from build123d import *

# Parameters (mm, degrees)
F1_DEPTH = 2
F2_R     = 1


with BuildPart() as f1:
    # F0 (on Top) → F1 (new body)
    with BuildSketch(Plane.XY):
        with BuildLine():
            ThreePointArc((13.617544, 3.25), (-14, 0), (13.617544, -3.25))
            Line((13.617544, -3.25), (2.436699, -1.75))
            ThreePointArc((2.436699, -1.75), (-3, 0), (2.436699, 1.75))
            Line((2.436699, 1.75), (13.617544, 3.25))
        make_face()
    extrude(amount=F1_DEPTH)

    # F2
    f2_edges = [f1.edges().sort_by_distance(p)[0] for p in [
        (13.617544, 3.25, 1),
        (13.617544, -3.25, 1),
    ]]
    fillet(f2_edges, radius=F2_R)


solid = f1.part
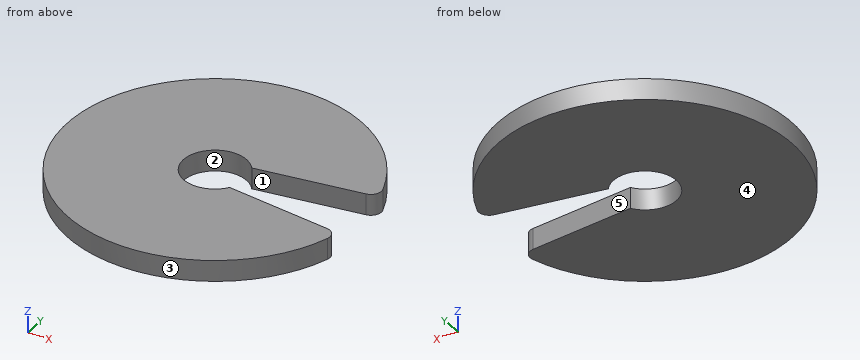
Build history of the part. All positions in model axes, mm. Face numbers are marked on the shaded views. A direction names the side the tool comes from. Give positions to 0.01 mm unless a question says otherwise; leave off trailing zeros. Loops run counter-clockwise (first coordinate to the right, second up) from the corner with the lowest first, then second, coordinate; pieces in that order, holes last. Notation, with made-up numbers: (-27, 27) - (-18, 27) arc R15 ccw to (-18, 43) - close; hole circle Ø4 at (72.25, 82). An arc over 180 degrees is marked (long way). Write item = value, one per line. Start each with the question number.
1) Band-saw the part on B-B on z = 1.2. Give the cut face in (x, y), plus the area to 3 significant figures.
2) Probe probe 1 along Y at (x, z) = (0, 1.4); probe 2 along Y at (x, z) = (3.25, 1.35); probe 3 along X at (y, z) = (4.25, 0.85). List the from-to ranges inside material, lowest first. Write a range as from..to.
3) Tool access for the marked faces 1 and 2: list every direction of +Z, -Z, +X, -X, +Y, -Y with a clear straight run to the whole face (end or side of a thin tool).
4) Drop flat-ended pins along their axis: pin 1 Ø1 at (y, z) = (3, 1.5) entering from +X; pin 2 Ø1 at (y, z) = (9.5, 1) entering from +X. Give the stop position or say it passes through.
5) Band-saw the part on C-C on x = 7.5. Give the cut face in (y, z), plus the area to 3 significant figures.
6) Pull direction Y, two halves, no side cores. Call the marked faces 3, 4 and 5: +Y half, -Y half, draft (parallel to the pull), parting line (faces both ways), or undercut.
7) Band-saw the part on A-A on x = 0. Give the cut face in (y, z).
8) Band-saw the part on D-D on y = 0. Give the cut face in (x, z).
Final values:
q1.outline = (2.44, -1.75) arc R3 cw (long way) to (2.44, 1.75) - (12.47, 3.1) arc R1 ccw to (13.29, 4.4) arc R14 ccw (long way) to (13.29, -4.4) arc R1 ccw to (12.47, -3.1) - close
q1.area = 531 mm²
q2.probe_1 = -14..-3, 3..14
q2.probe_2 = -13.62..-1.86, 1.86..13.62
q2.probe_3 = -13.34..13.33
q3.face_1 = +Z, -Z, +X
q3.face_2 = +Z, -Z
q4.pin_1 = 13.15
q4.pin_2 = 10.72
q5.outline = (-11.82, 0) - (-2.43, 0) - (-2.43, 2) - (-11.82, 2) - close; (2.43, 0) - (11.82, 0) - (11.82, 2) - (2.43, 2) - close
q5.area = 37.6 mm²
q6.face_3 = parting line
q6.face_4 = draft
q6.face_5 = undercut
q7.outline = (-14, 0) - (-3, 0) - (-3, 2) - (-14, 2) - close; (3, 0) - (14, 0) - (14, 2) - (3, 2) - close
q8.outline = (-14, 0) - (-3, 0) - (-3, 2) - (-14, 2) - close
